Can you work these out from the drawing? Everything is in mm from the part's minimum corner. A direction names the side the tool comes from. Coordinates: 2 decimals unless noted, no trailing zeros. Write each loop counter-clockwise with the first axis right and the second up, starting at its lowest first coordinate (ties: lowest second). Pieces come first, ordered by that corner, then holes.
(1) Which directions (+Z, -Z, +X, -X, +Y, -Y) give clear straight access to the entire face, cutting with the end or side of a thin tool? Please do the marked faces 4, 5 and 6.
(2) Imagine slicing it at D-D, the plane x = 2.5. List the corners of the cut face in (y, z) for me.
(3) Imagine slicing it at B-B, the plane y = 7.25. List the corners of the cut face in (x, z) for me.
(4) Thinking about a two-plate mould opening in Y: for the marked faces 1, 2 and 3, which applies, released by +Y, released by -Y, zero draft, split by the parting line, or undercut?
(5) Imagine slicing it at A-A, the plane x = 5.75. List the corners of the cut face in (y, z) for me.
(6) Please list where these lines run through material, in increasing order: probe 1 along Y at (x, z) = (5, 2.25); probe 2 along Z at (x, y) = (7.5, 8).
(7) Imagine slicing it at C-C, the plane z = 11.5. List the corners of the cut face in (x, y) for me, plus the area to 4 significant figures.
(8) For pin 1 Ø2.5 at (x, z) = (5, 16.5) entering from +Y; pin 2 Ø2 at (y, z) = (5.5, 14.5) entering from -X; pin 3 Ø3.5 at (y, z) = (3.5, 11.5) entering from +X, each with a flat end and sliding along its axis, tell me the tip position at first contact or that it passes through.
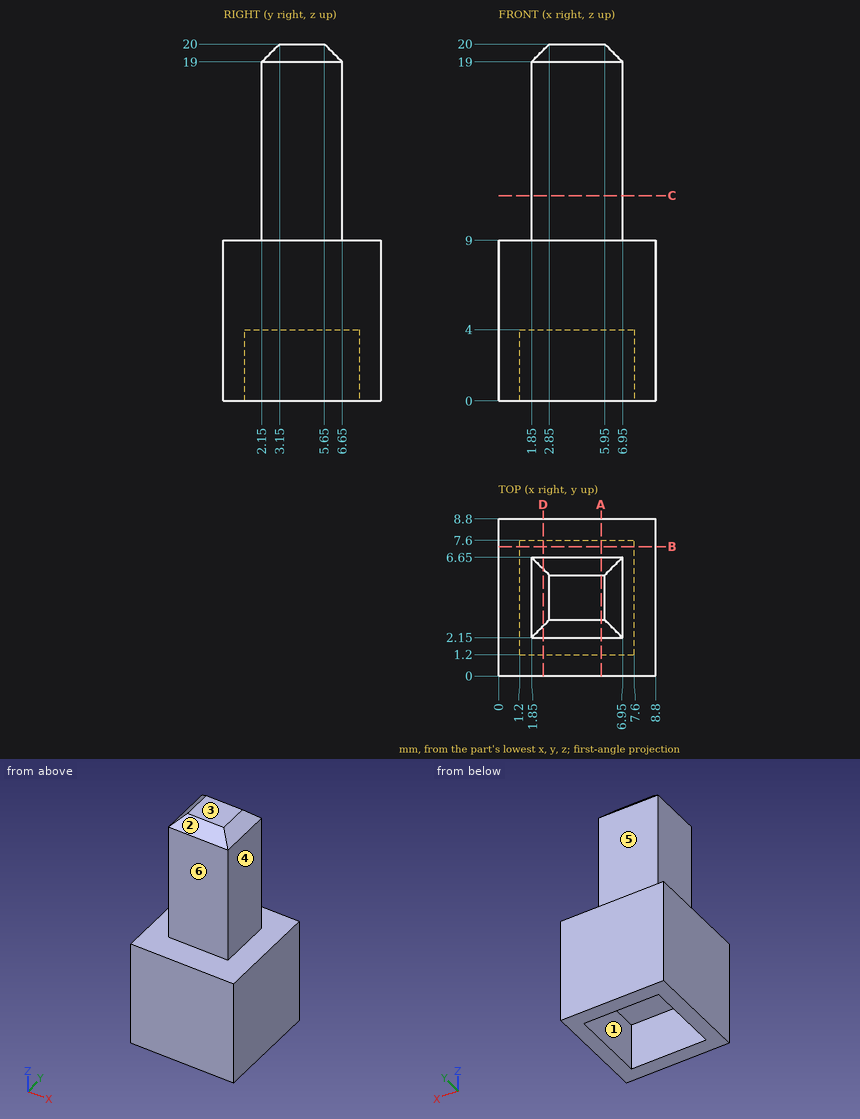
Recorded:
1. face 4: +Z, +X, +Y, -Y
1. face 5: +Z, +X, -X, +Y
1. face 6: +Z, +X, -X, -Y
2. outline: (0, 0) - (1.2, 0) - (1.2, 4) - (7.6, 4) - (7.6, 0) - (8.8, 0) - (8.8, 9) - (6.65, 9) - (6.65, 19) - (6, 19.65) - (2.8, 19.65) - (2.15, 19) - (2.15, 9) - (0, 9) - close
3. outline: (0, 0) - (1.2, 0) - (1.2, 4) - (7.6, 4) - (7.6, 0) - (8.8, 0) - (8.8, 9) - (0, 9) - close
4. face 1: undercut
4. face 2: released by -Y
4. face 3: zero draft
5. outline: (0, 0) - (1.2, 0) - (1.2, 4) - (7.6, 4) - (7.6, 0) - (8.8, 0) - (8.8, 9) - (6.65, 9) - (6.65, 19) - (5.65, 20) - (3.15, 20) - (2.15, 19) - (2.15, 9) - (0, 9) - close
6. probe 1: y = 0 to 1.2, 7.6 to 8.8
6. probe 2: z = 0 to 9
7. outline: (1.85, 2.15) - (6.95, 2.15) - (6.95, 6.65) - (1.85, 6.65) - close
7. area: 22.95 mm2
8. pin 1: stops at y = 6.65
8. pin 2: stops at x = 1.85
8. pin 3: stops at x = 6.95
